Could you check a few things on this model? Use its own coordinates, in mm. A direction names the side the tool comes from. Round coordinates to 2 decimals unless told otherwise and drop trailing zeros. Order: outer loops, then holes, each group sorted by start corner. A loop starts at its lowest first (then second) coordinate and runs counter-clockwise, first axis right, second up. Notation, with made-up numbers: (-24.75, 76.5) -> (33.25, 76.5) arc R16 ccw to (33.25, 92.5) -> close; hole circle Ø5 at (81.5, 10). An arc over 180 degrees is marked (long way). Put each result on its own line as item: value. Start each with the question number.
Autodesk Inventor part; units mm, degrees
ref_plane "c_k_XY" through (-4, 0, 0) normal (1, 0, 0) x (0, 0, -1)
ref_plane "c_k_YZ" through (-4, 0, 0) normal (0, 0, -1) x (0, 1, 0)
ref_plane "c_k_ZX" through (-4, 0, 0) normal (0, 1, 0) x (1, 0, 0)
sketch "Sketch_2" plane through (0, 0, 0) normal (0, 0, 1) x (1, 0, 0)
  line L0 (12, 0) -> (-8, 0)
  line L1 (-8, 12) -> (-8, 3)
  line L2 (-8, 3) -> (12, 3)
  line L3 (12, 3) -> (12, 8)
  line L4 (12, 8) -> (0, 8)
  line L5 (0, 8) -> (0, 12)
  line L6 (0, 12) -> (-8, 12)
revolve "Revolution1" add sketch "Sketch_2" angle 360 about axis through (12, 0, 0) along (1, 0, 0)
sketch "Sketch_4" plane through (0, 0, 0) normal (0, 0, 1) x (1, 0, 0)
  line L0 (6, 0) -> (6, 8)
  line L1 (6, 8) -> (7.5, 8)
  line L2 (7.5, 8) -> (7.2295, 7.7295)
  line L3 (7.2295, 7.7295) -> (7.2295, 0)
  line L4 (7.2295, 0) -> (6, 0)
  line L5 (6, 0) -> (6, 8)
revolve "Revolution2" cut sketch "Sketch_4" angle 360 about axis through (6, 0, 0) along (0, -1, 0)
sketch "Sketch_5" plane through (0, 0, 0) normal (0, 1, 0) x (-1, 0, 0)
  line L0 (-6, 0) -> (-6, -8)
  line L1 (-6, -8) -> (-7.5, -8)
  line L2 (-7.5, -8) -> (-7.2295, -7.7295)
  line L3 (-7.2295, -7.7295) -> (-7.2295, 0)
  line L4 (-7.2295, 0) -> (-6, 0)
  line L5 (-6, 0) -> (-6, -8)
revolve "Revolution3" cut sketch "Sketch_5" angle 360 about axis through (6, 0, 0) along (0, 0, 1)
thread "Thread1"
ref_plane "c_k_XY" through (-4, 0, 0) normal (1, 0, 0) x (0, 0, -1)
ref_plane "c_k_YZ" through (-4, 0, 0) normal (0, 0, -1) x (0, 1, 0)
ref_plane "c_k_ZX" through (-4, 0, 0) normal (0, 1, 0) x (1, 0, 0)
properties part number "UMHSL30_c"
1. For pin 1 Ø1 at (x, z) = (8, -4.5) entering from -Y; pin 2 Ø4 at (x, y) = (7.5, -2.5) entering from +Z; pin 3 Ø3 at (x, z) = (6, 0) entering from -Y, each with a flat end and sliding along its axis, tell me the tip position at first contact or that it passes through.
2. If we section it at B-B, the plane z = 0: Please give me the cut outline in (x, y), then the cut area to 3 significant figures.
3. Which directions (+Z, -Z, +X, -X, +Y, -Y) give clear straight access to the entire face, cutting with the end or side of a thin tool? Please do faces 4 (the face through (2.14, -2.21, 2.03)), 5 (the face through (7.136, -0.471, -5.198)), 6 (the face through (5.92, -1.73, 7.81)).
4. I need wall thicknesses on L1, parallel to X at y = 6.25, z = 0; L2, parallel to Z at x = -1.5, y = 0; L3, parallel to Z at x = 9.75, y = -2.75. Which ranges of each line are inside material? Lowest first, please.
5. If we section it at D-D, the plane x = 6: Please give me the cut outline in (y, z).
6. If we section it at A-A, the plane y = 0: Please give me the cut outline in (x, z), then the cut area to 3 significant figures.
7. Thinking about a two-plate mould opening in X: for faces 1 (the face through (-4.06, -11.99, -0.53)), 2 (the face through (7.136, 5.198, -0.471)), 3 (the face through (0, 2, -8)), which applies, +X half, -X half, draft (parallel to the pull), parting line (faces both ways), or undercut?
8. If we section it at C-C, the plane x = -0.5: Please give me the cut outline in (y, z), then the cut area to 3 significant figures.
Results below:
1. pin 1: y = -6.93
1. pin 2: z = 7.98
1. pin 3: y = -8
2. outline: (-8, -12) -> (0, -12) -> (0, -8) -> (12, -8) -> (12, -3) -> (-8, -3) -> close; (-8, 3) -> (4.77, 3) -> (4.77, 7.73) -> (4.5, 8) -> (0, 8) -> (0, 12) -> (-8, 12) -> close; (7.23, 3) -> (12, 3) -> (12, 8) -> (7.5, 8) -> (7.23, 7.73) -> close
2. area: 252 mm2
3. face 4: +X, -X
3. face 5: -Z
3. face 6: +X
4. L1: -8 to 4.77, 7.23 to 12
4. L2: -12 to -3, 3 to 12
4. L3: -7.51 to -1.2, 1.2 to 7.51
5. outline: (-1.38, -7.88) -> (-1.23, -7.73) -> (-1.23, -2.74) arc R3 cw (long way) to (2.74, 1.23) -> (7.73, 1.23) -> (7.88, 1.38) arc R8 ccw (long way) to start; (1.23, -7.73) -> (1.38, -7.88) arc R8 ccw to (7.88, -1.38) -> (7.73, -1.23) -> (2.74, -1.23) arc R3 cw to (1.23, -2.74) -> close
6. outline: (-8, -12) -> (0, -12) -> (0, -8) -> (4.5, -8) -> (4.77, -7.73) -> (4.77, -3) -> (-8, -3) -> close; (-8, 3) -> (12, 3) -> (12, 8) -> (0, 8) -> (0, 12) -> (-8, 12) -> close; (7.23, -7.73) -> (7.5, -8) -> (12, -8) -> (12, -3) -> (7.23, -3) -> close
6. area: 252 mm2
7. face 1: draft
7. face 2: undercut
7. face 3: +X half
8. outline: circle Ø24 at (0, 0); hole circle Ø6 at (0, 0)
8. area: 424 mm2
